Autodesk Inventor part; units mm, degrees
ref_plane "YZ Plane" through (0, 0, 0) normal (1, 0, 0) x (0, 1, 0)
ref_plane "XZ Plane" through (0, 0, 0) normal (0, 1, 0) x (-1, 0, 0)
ref_plane "XY Plane" through (0, 0, 0) normal (0, 0, 1) x (1, 0, 0)
sketch "Sketch1" plane through (0, 0, 0) normal (0, 1, 0) x (-1, 0, 0)
  circle A0 centre (15.7792, 0.2535) radius 2.1844 construction
  circle A1 centre (66.5792, 25.6535) radius 2.1844 construction
  circle A2 centre (66.5792, 12.9535) radius 2.1844 construction
  circle A3 centre (15.7792, -12.4465) radius 2.1844 construction
  circle A4 centre (15.7792, -12.4465) radius 2.3495
  circle A5 centre (15.7792, 0.2535) radius 2.3495
  circle A6 centre (66.5792, 12.9535) radius 2.3495
  circle A7 centre (66.5792, 25.6535) radius 2.3495
  line L0 (71.7164, -18.7965) -> (71.7164, 32.0035) construction
  arc A8 (71.7164, 25.6535) -> (64.3805, 30.2964) centre (66.5792, 25.6535) ccw
  arc A9 (9.4292, -12.4465) -> (22.0969, -13.0866) centre (15.7792, -12.4465) ccw
  line L1 (71.7164, 12.9535) -> (71.7164, 25.6535)
  line L2 (9.4292, -12.4465) -> (9.4292, 0.2535)
  line L3 (13.0614, 5.9925) -> (64.3805, 30.2964)
  line L4 (66.5792, 7.8164) -> (48.0123, 7.8164)
  line L5 (25.729, -2.0605) -> (45.2945, 7.2054)
  line L6 (22.0969, -13.0866) -> (22.0969, -7.7995)
  arc A10 (13.0614, 5.9925) -> (9.4292, 0.2535) centre (15.7792, 0.2535) ccw
  arc A11 (66.5792, 7.8164) -> (71.7164, 12.9535) centre (66.5792, 12.9535) ccw
  arc A12 (48.0123, 7.8164) -> (45.2945, 7.2054) centre (48.0123, 1.4664) ccw
  arc A13 (25.729, -2.0605) -> (22.0969, -7.7995) centre (28.4469, -7.7995) ccw
  point P0 (0, 0)
  dimension "d0" = 4.699
  dimension "d1" = 4.699
  dimension "d2" = 4.699
  dimension "d3" = 4.699
  dimension "d5" = 12.7
  dimension "d7" = 6.35
  dimension "d8" = 6.35
  dimension "d9" = 12.7
extrude "Plate1" add sketch "Sketch1" along normal blind 1.5875
equation "\"d10\" = Thickness"
equation "\"BendRadius\" = Thickness"
equation "\"BendReliefWidth\" = Thickness"
equation "\"BendReliefDepth\" = 0.5 * Thickness"
equation "\"CornerReliefSize\" = 4 * Thickness"
equation "\"MinimumRemnant\" = 2 * Thickness"
equation "\"TransitionRadius\" = BendRadius"
equation "\"JacobiRadiusSize\" = BendRadius"
equation "\"GapSize\" = Thickness"
properties part number "frontgussets"
The listing builds one solid part. Answer for the finished solid, in the listing's coordinates (mm). A direction names the side the tool comes from. Round coordinates to 2 decimals unless told otherwise and drop trailing zeros. Write each loop counter-clockwise with the first axis right and the second up, starting at its lowest first coordinate (ties: lowest second). Pieces come first, ordered by that corner, then holes. Notation, with made-up numbers: (48, 62.5) -> (82, 62.5) arc R19 ccw to (82, 95.5) -> close; hole circle Ø8 at (60.5, 82). An arc over 180 degrees is marked (long way). Use CSV: the item, a comma, the result in double quotes. Start each with the question number.
(1) Section C-C on z = -1 is taken. Give the vertices of the cut face in (x, y).
(2) Section A-A on y = 0.85 is taken. Give the vertices of the cut face in (x, z).
(3) Consider L1, parallel to X at y = 0.7, z = -12.5; L2, parallel to X at y = 0.4, z = -7.5; L3, parallel to Z at x = -17.5, y = 1.3. Determine where each line is inside the solid, lowest interval first. Write a range as from..to.
(4) Which of the six approach directions +Z, -Z, +X, -X, +Y, -Y give full straight-line access (tool end or side, diameter ignored) to faces 5 (the face through (-15.594, 0.783, -18.794)), 6 (the face through (-57, 1, 7.816))?
(5) Section B-B on x = -17 is taken. Give the vertices of the cut face in (y, z).
(6) The mould has two halves that part along Z. Classify faces 1 (the face through (-22.097, 1, -10)), 2 (the face through (-13.91, 0.78, -11.02)), 3 (the face through (-66.07, 0.783, 27.947)), 4 (the face through (-10.39, 0.78, 3.61)): released by +Z, released by -Z, zero draft, split by the parting line, or undercut.
(7) Section D-D on x = -67.5 is taken. Give the vertices of the cut face in (y, z), then the cut area to 3 significant figures.
A:
1,outline,"(-27.97, 0) -> (-17.77, 0) -> (-17.77, 1.59) -> (-27.97, 1.59) -> close; (-13.79, 0) -> (-9.43, 0) -> (-9.43, 1.59) -> (-13.79, 1.59) -> close"
2,outline,"(-71.72, 12.95) arc R5.14 ccw to (-66.58, 7.82) -> (-48.01, 7.82) arc R6.35 cw to (-45.29, 7.21) -> (-25.73, -2.06) arc R6.35 cw to (-22.1, -7.8) -> (-22.1, -13.09) arc R6.35 ccw to (-9.43, -12.45) -> (-9.43, 0.25) arc R6.35 ccw to (-13.06, 5.99) -> (-64.38, 30.3) arc R5.14 ccw to (-71.72, 25.65) -> close; hole circle Ø4.7 at (-66.58, 12.95); hole circle Ø4.7 at (-66.58, 25.65); hole circle Ø4.7 at (-15.78, -12.45); hole circle Ø4.7 at (-15.78, 0.25)"
3,L1,"x = -22.1..-18.13, -13.43..-9.43"
3,L2,"x = -22.1..-9.43"
3,L3,"z = -18.56..-14.05, -10.85..-1.35, 1.85..8.09"
4,face 5,"-Z, +Y, -Y"
4,face 6,"-Z, -X, +Y, -Y"
5,outline,"(0, -18.68) -> (1.59, -18.68) -> (1.59, -14.45) -> (0, -14.45) -> close; (0, -10.44) -> (1.59, -10.44) -> (1.59, -1.75) -> (0, -1.75) -> close; (0, 2.26) -> (1.59, 2.26) -> (1.59, 7.86) -> (0, 7.86) -> close"
6,face 1,"zero draft"
6,face 2,"undercut"
6,face 3,"undercut"
6,face 4,"released by +Z"
7,outline,"(0, 7.9) -> (1.59, 7.9) -> (1.59, 10.79) -> (0, 10.79) -> close; (0, 15.12) -> (1.59, 15.12) -> (1.59, 23.49) -> (0, 23.49) -> close; (0, 27.82) -> (1.59, 27.82) -> (1.59, 30.71) -> (0, 30.71) -> close"
7,area,"22.5 mm²"
